```python
from build123d import *

# Parameters (mm, degrees)
SKETCH1_R           = 12.7
BOSS_EXTRUDE1_DEPTH = 6.35
CUT_EXTRUDE1_DEPTH  = 3.175
SKETCH1_5_R         = 1.193106662
CUT_EXTRUDE2_DEPTH  = 20.05


with BuildPart() as part:
    # Sketch1 → Boss-Extrude1 (new body)
    with BuildSketch(Plane(origin=(0, 0, 0), x_dir=(1, 0, 0), z_dir=(0, 1, 0))):
        with Locations(Location((0, 0, 0), (0, 0, 270))):
            Circle(SKETCH1_R)
    extrude(amount=BOSS_EXTRUDE1_DEPTH)

    # Sketch1_3 → Cut-Extrude1 (cut)
    with BuildSketch(Plane(origin=(0, 0, 0), x_dir=(1, 0, 0), z_dir=(0, 1, 0))):
        with BuildLine():
            ThreePointArc((-9.498704201, 0.707278937), (-9.326008306, 0.372216353), (-9.26646174, 0))
            Line((-9.26646174, 0), (9.26646174, 0))
            ThreePointArc((9.26646174, 0), (9.326008306, 0.372216353), (9.498704201, 0.707278937))
            ThreePointArc((9.498704201, 0.707278937), (0, 9.525), (-9.498704201, 0.707278937))
        make_face()
        with BuildLine():
            Line((9.26646174, 0), (-9.26646174, 0))
            ThreePointArc((-9.26646174, 0), (-9.326008306, -0.372216353), (-9.498704201, -0.707278937))
            ThreePointArc((-9.498704201, -0.707278937), (0, -9.525), (9.498704201, -0.707278937))
            ThreePointArc((9.498704201, -0.707278937), (9.326008306, -0.372216353), (9.26646174, 0))
        make_face()
    extrude(amount=CUT_EXTRUDE1_DEPTH, mode=Mode.SUBTRACT)

    # Sketch1_5 → Cut-Extrude2 (cut, through all)
    with BuildSketch(Plane(origin=(0, 0, 0), x_dir=(1, 0, 0), z_dir=(0, 1, 0))):
        with Locations(Location((-10.459568402, 0, 0), (0, 0, 36.356273959))):
            Circle(SKETCH1_5_R)
        with Locations(Location((10.459568402, 0, 0), (0, 0, 143.643726041))):
            Circle(SKETCH1_5_R)
    extrude(amount=CUT_EXTRUDE2_DEPTH, mode=Mode.SUBTRACT)


solid = part.part
```
Geometry: final body of the model. Coordinates: model frame, mm. A direction names the side the tool comes from. Round coordinates to 2 decimals unless told otherwise and drop trailing zeros. Write each loop counter-clockwise with the first axis right and the second up, starting at its lowest first coordinate (ties: lowest second). Pieces come first, ordered by that corner, then holes.
Item 1: Section query C-C (y = 3.5). Return loops of the section in (x, z), plus the area to 3 significant figures.
Item 2: Mould query, pull axis Z, two halves, no side actions, for faces 3 (the face through (-9.3, 0, 2.8)), 4 (the face through (-7.7, 3.1, -10.1)), 5 (the face through (11.652, 3.131, -0.023)). Classes: +Z half, -Z half, draft (parallel to the pull), parting line (faces both ways), or undercut.
Item 3: Section query A-A (z = 0). Return loops of the section in (x, y) (3 decimals).
Item 4: Pin query (flat end, axial travel): P1, Ø1.9, axis at x = 10.46, z = 0, coming from the -Y side; P2, Ø1, axis at x = 0.5, z = -3.5, coming from the -Y side (3 decimals); P3, Ø3, axis at x = -4.5, y = 2.5, coming from the +Z side. Return the tip coordinate at first contact, or that it passes through.
Item 5: Section query D-D (x = 0). Return loops of the section in (y, z) (3 decimals), plus the area to 3 significant figures.
Item 6: Section query B-B (x = 10.75). Return loops of the section in (y, z), plus the area to 3 significant figures.
Item 7: Set-up query: faces 1 (the face through (0, 3.175, 0)), 2 (the face through (0, 6.35, 0)). Return all of +Z, -Z, +X, -X, +Y, -Y with unobstructed straight access to the full face (end or side cutting, diameter ignored); none if empty.
Item 8: Material intervals for L1, parallel to X at y = 3.25, z = 0; L2, parallel to X at y = 2.25, z = 0; L3, parallel to Y at x = -6.5, z = 1.75 (3 decimals), sorted ascending.
Completed:
1. outline: circle Ø25.4 at (0, 0); hole circle Ø2.39 at (-10.46, 0); hole circle Ø2.39 at (10.46, 0)
1. area: 498 mm2
2. face 3: draft
2. face 4: parting line
2. face 5: undercut
3. outline: (-12.7, 0) - (-11.653, 0) - (-11.653, 6.35) - (-12.7, 6.35) - close; (-9.266, 3.175) - (9.266, 3.175) - (9.266, 6.35) - (-9.266, 6.35) - close; (11.653, 0) - (12.7, 0) - (12.7, 6.35) - (11.653, 6.35) - close
4. P1: passes through
4. P2: stops at y = 3.175
4. P3: stops at z = 12.34
5. outline: (0, -12.7) - (6.35, -12.7) - (6.35, 12.7) - (0, 12.7) - (0, 9.525) - (3.175, 9.525) - (3.175, -9.525) - (0, -9.525) - close
5. area: 101 mm2
6. outline: (0, -6.76) - (6.35, -6.76) - (6.35, -1.16) - (0, -1.16) - close; (0, 1.16) - (6.35, 1.16) - (6.35, 6.76) - (0, 6.76) - close
6. area: 71.2 mm2
7. face 1: -Y
7. face 2: +Z, -Z, +X, -X, +Y
8. L1: x = -12.7 to -11.65, -9.27 to 9.27, 11.65 to 12.7
8. L2: x = -12.7 to -11.65, 11.65 to 12.7
8. L3: y = 3.175 to 6.35
